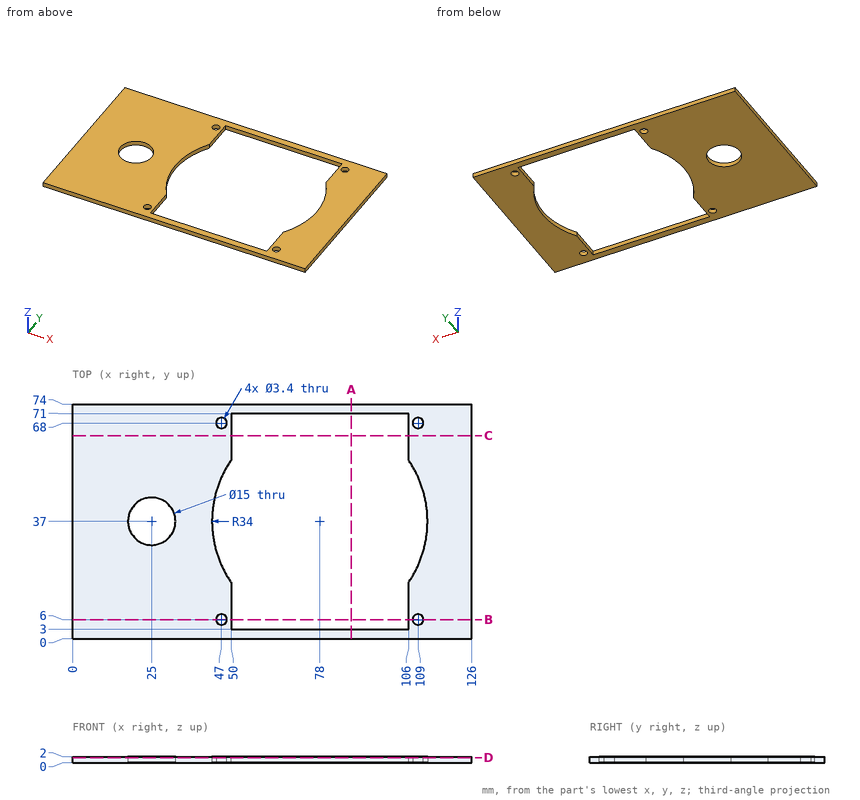
Can you work these out from the drawing? Everything is in mm from the part's minimum corner. Coordinates: 2 decimals unless noted, no trailing zeros. Loops run counter-clockwise (first coordinate to the right, second up) from the corner with the lowest first, then second, coordinate; pieces in that order, holes last. Notation, with made-up numbers: M 84.5,61 L 140.5,61 A34 ccw 140.5,92 Z; hole C 87,71.5 d5. An arc over 180 degrees is marked long. Put each result on its own line as item: value. Start each with the question number.
(1) I need wall thicknesses on line 1 (X direction, y = 6, z = 1.15); line 2 (X direction, y = 65, z = 1.7); line 3 (Y direction, x = 95.5, z = 0.9). Which ranges of each line are inside material? Lowest first, please. Write a range as from..to.
(2) Suppose I cut it at C-C on y = 64. Please give me the cut outline in (x, z), then the cut area to 3 significant figures.
(3) Suppose I cut it at A-A on x = 88. Please give me the cut outline in (y, z).
(4) Suppose I cut it at B-B on y = 6. Please give me the cut outline in (x, z).
(5) Suppose I cut it at D-D on z = 1.7. Please give me the cut outline in (x, y).
Solutions:
1. line 1: x = 0..45.3, 48.7..50, 106..107.3, 110.7..126
1. line 2: x = 0..50, 106..126
1. line 3: y = 0..3, 71..74
2. outline: M 0,0 L 50,0 L 50,2 L 0,2 Z; M 106,0 L 126,0 L 126,2 L 106,2 Z
2. area: 140 mm2
3. outline: M 0,0 L 3,0 L 3,2 L 0,2 Z; M 71,0 L 74,0 L 74,2 L 71,2 Z
4. outline: M 0,0 L 45.3,0 L 45.3,2 L 0,2 Z; M 48.7,0 L 50,0 L 50,2 L 48.7,2 Z; M 106,0 L 107.3,0 L 107.3,2 L 106,2 Z; M 110.7,0 L 126,0 L 126,2 L 110.7,2 Z
5. outline: M 0,0 L 126,0 L 126,74 L 0,74 Z; hole C 25,37 d15; hole C 47,6 d3.4; hole C 47,68 d3.4; hole M 50,3 L 106,3 L 106,17.71 A34 ccw 106,56.29 L 106,71 L 50,71 L 50,56.29 A34 ccw 50,17.71 Z; hole C 109,6 d3.4; hole C 109,68 d3.4
